Part model, mm, in its own coordinate system. Face numbers are marked on the shaded views. A direction names the side the tool comes from. Round coordinates to 2 decimals unless told otherwise and drop trailing zeros. Loops run counter-clockwise (first coordinate to the right, second up) from the corner with the lowest first, then second, coordinate; pieces in that order, holes last.
(1) Mould opens along X. For the marked faces 4, 5 and 6 say: +X half, -X half, draft (parallel to the pull), parting line (faces both ways), or undercut.
(2) Cut at A-A on z = 2.25. List the corners of the cut face in (x, y).
(3) Cut at D-D on x = -10. List the corners of the cut face in (y, z), then the cut area to 3 significant figures.
(4) Tool access for the marked faces 1, 2 and 3: list every direction of +Z, -Z, +X, -X, +Y, -Y with a clear straight run to the whole face (end or side of a thin tool).
(5) Cut at C-C on x = 0. List the corners of the cut face in (y, z), then the cut area to 3 significant figures.
(6) Probe probe 1 along Y at (x, z) = (0, 5.75); probe 2 along X at (y, z) = (4.25, 5); probe 3 along Y at (x, z) = (-4, 4.5). List the from-to ranges inside material, lowest first.
(7) Flat gauge pins, fed straight in: pin 1 (1.5 mm diameter, centred on x = 11.5, y = -3, fed in from -Z); pin 2 (4 mm diameter, centred on x = 7.89, y = 0, fed in from +Z); pin 3 (5.5 mm diameter, centred on x = 7.5, y = -0.5, fed in from -Z). Where does each tip first touch, or does it go through?
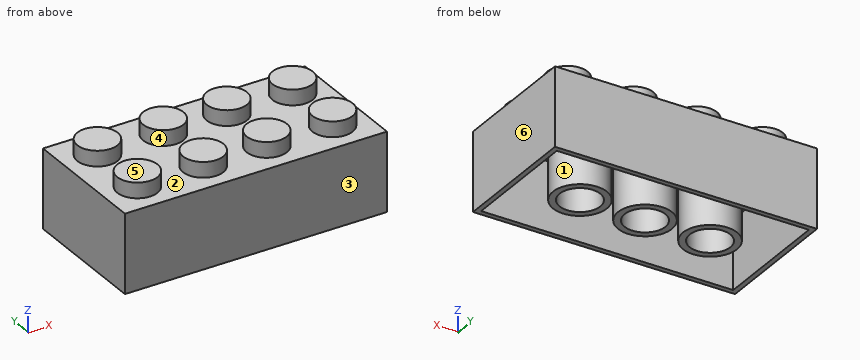
from build123d import *

# Parameters (mm, degrees)
F0_W      = 31.7754
F0_H      = 15.8369
F1_DEPTH  = 9.5377
F2_R      = 2.44475
F3_DEPTH  = 1.8669
F5_W      = 30.5689
F5_H      = 14.6304
F6_DEPTH  = 8.382
F7_R      = 3.27025
F8_DEPTH  = 8.382
F9_R      = 2.47015
F10_DEPTH = 8.382


with BuildPart() as f1:
    # F0 (on Top) → F1 (new body)
    with BuildSketch(Plane.XY):
        Rectangle(F0_W, F0_H)
    extrude(amount=F1_DEPTH)

    # F2 (on face) → F3 (join)
    with BuildSketch(Plane.XY.offset(9.5377)):
        with Locations((-11.83005, 3.8608)):
            Circle(F2_R)
        with Locations((-3.85445, 3.8608)):
            Circle(F2_R)
        with Locations((3.85445, 3.8608)):
            Circle(F2_R)
        with Locations((11.83005, 3.8608)):
            Circle(F2_R)
        with Locations((-11.83005, -3.8608)):
            Circle(F2_R)
        with Locations((-3.85445, -3.8608)):
            Circle(F2_R)
        with Locations((3.85445, -3.8608)):
            Circle(F2_R)
        with Locations((11.83005, -3.8608)):
            Circle(F2_R)
    extrude(amount=F3_DEPTH)

    # F5 (on plane+point) → F6 (cut)
    with BuildSketch(Plane(origin=(0, 0, 0), x_dir=(1, 0, 0), z_dir=(0, 0, -1))):
        Rectangle(F5_W, F5_H)
    extrude(amount=-F6_DEPTH, mode=Mode.SUBTRACT)

    # F7 (on face) → F8 (join)
    with BuildSketch(Plane(origin=(0, 0, 8.382), x_dir=(1, 0, 0), z_dir=(0, 0, -1))):
        with Locations((-7.8867, 0)):
            Circle(F7_R)
        Circle(F7_R)
        with Locations((7.8867, 0)):
            Circle(F7_R)
    extrude(amount=F8_DEPTH)

    # F9 (on face) → F10 (cut)
    with BuildSketch(Plane(origin=(0, 0, 0), x_dir=(1, 0, 0), z_dir=(0, 0, -1))):
        with Locations((-7.8867, 0)):
            Circle(F9_R)
        Circle(F9_R)
        with Locations((7.8867, 0)):
            Circle(F9_R)
    extrude(amount=-F10_DEPTH, mode=Mode.SUBTRACT)


solid = f1.part
Final values:
1. face 4: undercut
1. face 5: draft
1. face 6: +X half
2. outline: (-15.89, -7.92) - (15.89, -7.92) - (15.89, 7.92) - (-15.89, 7.92) - close; circle Ø6.54 at (-7.89, 0); circle Ø6.54 at (0, 0); circle Ø6.54 at (7.89, 0); hole (-15.28, -7.32) - (15.28, -7.32) - (15.28, 7.32) - (-15.28, 7.32) - close; hole circle Ø4.94 at (-7.89, 0); hole circle Ø4.94 at (0, 0); hole circle Ø4.94 at (7.89, 0)
3. outline: (-7.92, 0) - (-7.32, 0) - (-7.32, 8.38) - (-2.5, 8.38) - (-2.5, 0) - (-1.28, 0) - (-1.28, 8.38) - (1.28, 8.38) - (1.28, 0) - (2.5, 0) - (2.5, 8.38) - (7.32, 8.38) - (7.32, 0) - (7.92, 0) - (7.92, 9.54) - (5.48, 9.54) - (5.48, 11.4) - (2.24, 11.4) - (2.24, 9.54) - (-2.24, 9.54) - (-2.24, 11.4) - (-5.48, 11.4) - (-5.48, 9.54) - (-7.92, 9.54) - close
3. area: 60.9 mm2
4. face 1: -Z
4. face 2: +Z
4. face 3: +Z, -Z, +X, -X, -Y
5. outline: (-7.92, 0) - (-7.32, 0) - (-7.32, 8.38) - (-3.27, 8.38) - (-3.27, 0) - (-2.47, 0) - (-2.47, 8.38) - (2.47, 8.38) - (2.47, 0) - (3.27, 0) - (3.27, 8.38) - (7.32, 8.38) - (7.32, 0) - (7.92, 0) - (7.92, 9.54) - (-7.92, 9.54) - close
5. area: 41.8 mm2
6. probe 1: y = -7.92 to -7.32, -3.27 to -2.47, 2.47 to 3.27, 7.32 to 7.92
6. probe 2: x = -15.89 to -15.28, 15.28 to 15.89
6. probe 3: y = -7.92 to -7.32, 7.32 to 7.92
7. pin 1: stops at z = 8.38
7. pin 2: stops at z = 9.54
7. pin 3: stops at z = 0
